Geometry check sheet. Reference: the model listing, model coordinates, mm. Face numbers are marked on the shaded views. A direction names the side the tool comes from. Give positions to 0.01 mm unless a question says otherwise; leave off trailing zeros. Loops run counter-clockwise (first coordinate to the right, second up) from the corner with the lowest first, then second, coordinate; pieces in that order, holes last. Notation, with made-up numbers: (30.25, 87) -> (84.25, 87) arc R7 cw to (84.25, 94) -> close; hole circle Ø5 at (15, -31). An arc over 180 degrees is marked (long way). Write item = value, one per line.
Autodesk Inventor part; units mm, degrees
ref_plane "YZ Plane" through (0, 0, 0) normal (1, 0, 0) x (0, 1, 0)
ref_plane "XZ Plane" through (0, 0, 0) normal (0, 1, 0) x (-1, 0, 0)
ref_plane "XY Plane" through (0, 0, 0) normal (0, 0, 1) x (1, 0, 0)
sketch "Sketch1" plane through (0, 0, 0) normal (0, 0, 1) x (1, 0, 0)
  line L0 (-21.2649, 0) -> (21.2649, 0)
  line L1 (0, -30.5308) -> (0, 22.8092)
  arc A0 (15.1892, 0) -> (-15.1892, 0) centre (0, 0) ccw
  line L2 (-15.1892, 0) -> (15.1892, 0)
  line L3 (15.1892, 0) -> (15.1892, -22.9108)
  line L4 (15.1892, -22.9108) -> (-15.1892, -22.9108)
  line L5 (-15.1892, -22.9108) -> (-15.1892, 0)
  dimension "d0" = 30.3784
  dimension "d1" = 38.1
extrude "Extrusion1" add sketch "Sketch1" along normal blind 12.7
sketch "Sketch2" plane through (0, 0, 12.7) normal (0, 0, 1) x (1, 0, 0)
  arc A0 (15.1892, 0) -> (-15.1892, 0) centre (0, 0) ccw
  circle A1 centre (0, 0) radius 4.7625
  dimension "d4" = 9.525
extrude "Extrusion2" add sketch "Sketch2" along normal blind 7.5438
sketch "Sketch3" plane through (0, 0, 20.2438) normal (0, 0, 1) x (1, 0, 0)
  circle A0 centre (0, 0) radius 4.7625
  circle A1 centre (0, 0) radius 3.175
  dimension "d7" = 6.35
extrude "Extrusion3" add sketch "Sketch3" along normal blind 12.6492 contours A1
thread "Thread1"
sketch "Sketch4" plane through (-15.1892, -22.9108, 0) normal (0, -1, 0) x (1, 0, 0)
  line L0 (30.3784, 12.7) -> (0, 12.7)
  line L1 (0, 0) -> (0, 12.7)
  line L2 (10.033, 9.525) -> (10.8267, 9.525)
  line L3 (10.8267, 9.525) -> (10.8267, 8.7313)
  line L4 (10.8267, 8.7313) -> (10.033, 8.7313)
  line L5 (10.033, 8.7313) -> (10.033, 9.525)
  line L6 (13.208, 9.525) -> (14.0017, 9.525)
  line L7 (14.0017, 9.525) -> (14.0017, 8.7313)
  line L8 (14.0017, 8.7313) -> (13.208, 8.7313)
  line L9 (13.208, 8.7313) -> (13.208, 9.525)
  line L10 (16.383, 9.525) -> (17.1767, 9.525)
  line L11 (17.1767, 9.525) -> (17.1767, 8.7313)
  line L12 (17.1767, 8.7313) -> (16.383, 8.7313)
  line L13 (16.383, 8.7313) -> (16.383, 9.525)
  line L14 (19.558, 9.525) -> (20.3517, 9.525)
  line L15 (20.3517, 9.525) -> (20.3517, 8.7313)
  line L16 (20.3517, 8.7313) -> (19.558, 8.7313)
  line L17 (19.558, 8.7313) -> (19.558, 9.525)
  point P0 (15.1892, 0)
  dimension "d12" = 0.7937
  dimension "d13" = 10.033
  dimension "d14" = 3.175
  dimension "d17" = 3.175
extrude "Pins" add sketch "Sketch4" along normal blind 9.525
properties part number "encoder"
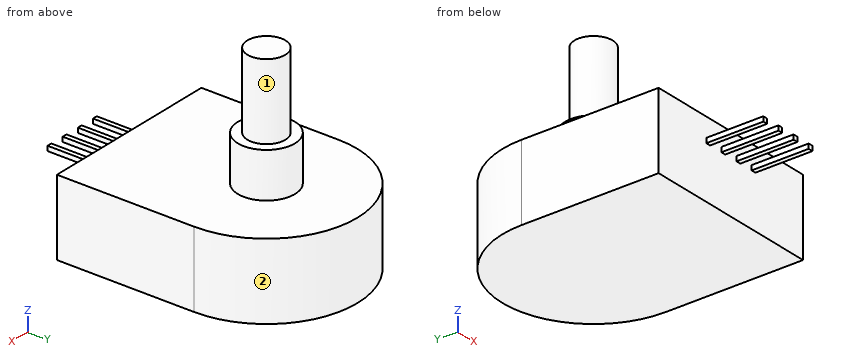
Item 1: Section check C-C, the plane y = -2. Record the cut outline in (x, z).
Answer:
outline = (-15.19, 0) -> (15.19, 0) -> (15.19, 12.7) -> (4.32, 12.7) -> (4.32, 20.24) -> (2.47, 20.24) -> (2.47, 32.89) -> (-2.47, 32.89) -> (-2.47, 20.24) -> (-4.32, 20.24) -> (-4.32, 12.7) -> (-15.19, 12.7) -> close
Item 2: Tool access check on the marked faces 1 and 2. Record the directions out of +Z, -Z, +X, -X, +Y, -Y that give a thin tool (end or side, any length) a straight path to the whole face; none if there is none.
Answer:
face_1 = +Z
face_2 = +Z, -Z, +Y
Item 3: Thickness scan on L1, parallel to Z at x = 13, y = -9.5; L2, parallel to Y at x = -1.5, z = 23.5; L3, parallel to Y at x = 10, z = 6.5. Record the ranges inside material, lowest first. Write a range as [from, to].
Answer:
L1 = [0, 12.7]
L2 = [-2.8, 2.8]
L3 = [-22.91, 11.43]
Item 4: Section check B-B, the plane z = 19. Record the cut outline in (x, y) (1 decimal).
Answer:
outline = circle Ø9.5 at (0, 0)
Item 5: Section check A-A, the plane x = 0. Record the cut outline in (y, z) (1 decimal), plus the area to 3 significant figures.
Answer:
outline = (-22.9, 0) -> (15.2, 0) -> (15.2, 12.7) -> (4.8, 12.7) -> (4.8, 20.2) -> (3.2, 20.2) -> (3.2, 32.9) -> (-3.2, 32.9) -> (-3.2, 20.2) -> (-4.8, 20.2) -> (-4.8, 12.7) -> (-22.9, 12.7) -> close
area = 636 mm^2
Item 6: Section check D-D, the plane z = 10.5. Record the cut outline in (x, y), plus the area to 3 significant figures.
Answer:
outline = (-15.19, -22.91) -> (15.19, -22.91) -> (15.19, 0) arc R15.19 ccw to (-15.19, 0) -> close
area = 1,060 mm^2
Item 7: Gauge pin test, flat ends, axial feed: pin 1 (0.6 mm diameter, centred on y = -30, z = 9, fed in from -X); pin 2 (0.9 mm diameter, centred on y = -26.5, z = 9.5, fed in from +X); pin 3 (0.6 mm diameter, centred on x = -4.5, y = -26, fed in from +Z) (3 decimals). Record the tip position at first contact, or that the pin passes through.
Answer:
pin_1 = -5.16
pin_2 = 5.16
pin_3 = 9.525
